For this review, take the finished solid that the model builds, in its own axes (mm). A direction names the side the tool comes from. Give positions to 0.01 mm unless a question says otherwise; leave off trailing zeros. Loops run counter-clockwise (first coordinate to the right, second up) from the corner with the lowest first, then second, coordinate; pieces in that order, holes last. Notation, with made-up numbers: (27.25, 69) -> (64.25, 69) arc R17 cw to (64.25, 76) -> close; hole circle Ø5 at (33.25, 61.5). An arc over 180 degrees is marked (long way). Answer as CSV lines item,"result". Start each with the question number.
Item 1: The part is to be moulded in two halves that separate along Y. For faces 1 (the face through (-6, -27.695, 57)), 2 (the face through (0, -41, 48.58)), 3 (the face through (5, -29.195, 35)), say which applies: +Y half, -Y half, draft (parallel to the pull), parting line (faces both ways), or undercut.
Item 2: Machinability: for faces 4 (the face through (0, -54.195, 69)), 5 (the face through (-6, -13.445, 6)), 6 (the face through (5, -29.195, 69)), which of the approach directions +Z, -Z, +X, -X, +Y, -Y give a long, thin tool a straight path to every point of the face, cutting with its end or side? Answer none if there is none.
Item 3: Clearance check with flat-ended pins moving along their axes: P1, Ø4.5, axis at y = 16.5, z = 34.5, coming from the +X side; P2, Ø5, axis at y = 9.5, z = 65.5, coming from the +X side; P3, Ø21, axis at y = 1.86, z = 46.03, coming from the +X side. State where each tip first meets the part, or that it passes through.
Item 4: Add section B-B on z = 12. State the section outline as (x, y) points, plus the area to 3 significant figures.
Item 5: Add section A-A on z = 46.03. State the section outline as (x, y) points.
Item 6: Add section C-C on y = -10. State the section outline as (x, z) points.
Item 7: Add section D-D on y = 25.5. State the section outline as (x, z) points, plus the area to 3 significant figures.
Item 8: For L1, parallel to Y at x = -1.25, z = 33; L2, parallel to Z at x = -7.5, y = -44.5; L3, parallel to Z at x = -2, y = -33.5, list the stretches that pass through material, from the lowest coordinate up. Write a range as from..to.
```python
from build123d import *

# Parameters (mm, degrees)
PROFILEEXTRUDE_DEPTH    = 73.76
HOSEWINDOW_W            = 16.29
HOSEWINDOW_H            = 26.5
HOSEWINDOWCUT_DEPTH     = 23.11
CAGESCREWS_R            = 2.4
CAGESCREWSCUT_DEPTH     = 23.11
AXLEHOLECUT_DEPTH       = 23.11
SETSCREWHOLES_R         = 1.539432213
SETSCREWHOLES_R_2       = 1.628953018
SETSCREWHOLESCUT_DEPTH  = 23.11
VELOCITYWINDOW_W        = 12.61
VELOCITYWINDOW_H        = 22.29
VELOCITYWINDOWCUT_DEPTH = 23.11
FILLET3_R               = 7
TRIGGERRACKSLOTCUT_W    = 6.7
TRIGGERRACKSLOTCUT_H    = 6.7
RACKSLOTCUT_DEPTH       = 23.11
FILLET4_R               = 1


with BuildPart() as part:
    # Profile → ProfileExtrude (new body)
    with BuildSketch(Plane.XY):
        with BuildLine():
            Line((10.261269376, -54.194713793), (10.261269376, -29.194713793))
            Line((10.261269376, -29.194713793), (-0.848730624, -29.194713793))
            Line((-0.848730624, -29.194713793), (-0.848730624, -13.194713793))
            ThreePointArc((-0.848730624, -13.194713793), (-4.204080189, -9.618555822), (-6.340730624, -5.204713793))
            Line((-6.340730624, -5.204713793), (-8.928730624, -5.204713793))
            Line((-8.928730624, -5.204713793), (-8.928730624, 6.495286207))
            Line((-8.928730624, 6.495286207), (-6.509650624, 6.495286207))
            ThreePointArc((-6.509650624, 6.495286207), (-4.40075771, 10.230064383), (-1.388730624, 13.283536207))
            Line((-1.388730624, 13.283536207), (-1.388730624, 21.845286207))
            Line((-1.388730624, 21.845286207), (10.261269376, 21.845286207))
            Line((10.261269376, 21.845286207), (10.261269376, 31.845286207))
            Line((10.261269376, 31.845286207), (-11.848730624, 31.845286207))
            Line((-11.848730624, 31.845286207), (-11.848730624, -54.194713793))
            Line((-11.848730624, -54.194713793), (10.261269376, -54.194713793))
        make_face()
    extrude(amount=PROFILEEXTRUDE_DEPTH)

    # HoseWindow → HoseWindowCut (cut, through all)
    with BuildSketch(Plane.ZY.offset(11.848730624)):
        with Locations((56.725, -40.944713793)):
            Rectangle(HOSEWINDOW_W, HOSEWINDOW_H)
    extrude(amount=-HOSEWINDOWCUT_DEPTH, mode=Mode.SUBTRACT)

    # CageScrews → CageScrewsCut (cut, through all)
    with BuildSketch(Plane.ZY.offset(11.848730624)):
        with Locations((7.5, 26.845286207)):
            Circle(CAGESCREWS_R)
        with Locations((66.26, 26.845286207)):
            Circle(CAGESCREWS_R)
        with Locations((7.5, -49.194713793)):
            Circle(CAGESCREWS_R)
        with Locations((69.31, -49.194713793)):
            Circle(CAGESCREWS_R)
    extrude(amount=-CAGESCREWSCUT_DEPTH, mode=Mode.SUBTRACT)

    # AxleHole → AxleHoleCut (cut, through all)
    with BuildSketch(Plane.ZY.offset(11.848730624)):
        with BuildLine():
            Line((47.361, 8.359497151), (47.361, 6.740497151))
            Line((47.361, 6.740497151), (44.699, 6.740497151))
            Line((44.699, 6.740497151), (44.699, 8.359497151))
            ThreePointArc((44.699, 8.359497151), (46.03, -4.783713793), (47.361, 8.359497151))
        make_face()
    extrude(amount=-AXLEHOLECUT_DEPTH, mode=Mode.SUBTRACT)

    # SetScrewHoles → SetScrewHolesCut (cut, through all)
    with BuildSketch(Plane.ZY.offset(11.848730624)):
        with Locations((6.03, 1.855286207)):
            Circle(SETSCREWHOLES_R)
        with Locations((68.03, 1.855286207)):
            Circle(SETSCREWHOLES_R_2)
    extrude(amount=-SETSCREWHOLESCUT_DEPTH, mode=Mode.SUBTRACT)

    # VelocityWindow → VelocityWindowCut (cut, through all)
    with BuildSketch(Plane.ZY.offset(11.848730624)):
        with Locations((32.655, -15.499713793)):
            Rectangle(VELOCITYWINDOW_W, VELOCITYWINDOW_H)
    extrude(amount=-VELOCITYWINDOWCUT_DEPTH, mode=Mode.SUBTRACT)

    # Fillet3
    fillet3_edges = [part.edges().sort_by_distance(p)[0] for p in [
        (-11.848730624, -26.644713793, 32.655),
    ]]
    fillet(fillet3_edges, radius=FILLET3_R)

    # TriggerRackSlotCut → RackSlotCut (cut, through all)
    with BuildSketch(Plane.ZY.offset(11.848730624)):
        with Locations((18.35, -44.494713793)):
            Rectangle(TRIGGERRACKSLOTCUT_W, TRIGGERRACKSLOTCUT_H)
        with Locations((30.95, -44.494713793)):
            Rectangle(TRIGGERRACKSLOTCUT_W, TRIGGERRACKSLOTCUT_H)
        with Locations((5.75, -31.794713793)):
            Rectangle(TRIGGERRACKSLOTCUT_W, TRIGGERRACKSLOTCUT_H)
        with Locations((18.35, -31.794713793)):
            Rectangle(TRIGGERRACKSLOTCUT_W, TRIGGERRACKSLOTCUT_H)
        with Locations((5.75, -16.794713793)):
            Rectangle(TRIGGERRACKSLOTCUT_W, TRIGGERRACKSLOTCUT_H)
        with Locations((18.35, -16.794713793)):
            Rectangle(TRIGGERRACKSLOTCUT_W, TRIGGERRACKSLOTCUT_H)
    extrude(amount=-RACKSLOTCUT_DEPTH, mode=Mode.SUBTRACT)

    # Fillet4
    fillet4_edges = [part.edges().sort_by_distance(p)[0] for p in [
        (-11.848730624, -11.174713793, 73.76),
        (-11.848730624, -18.999713793, 26.35),
        (-11.848730624, -18.999713793, 38.96),
        (-11.848730624, -4.354713793, 32.655),
        (-11.848730624, -44.494713793, 15),
        (-11.848730624, -47.844713793, 18.35),
        (-11.848730624, -44.494713793, 21.7),
        (-11.848730624, -41.144713793, 18.35),
        (-11.848730624, -11.174713793, 0),
        (-11.848730624, -44.494713793, 27.6),
        (-11.848730624, -47.844713793, 30.95),
        (-11.848730624, -44.494713793, 34.3),
        (-11.848730624, -41.144713793, 30.95),
        (-11.848730624, -31.794713793, 2.4),
        (-11.848730624, -35.144713793, 5.75),
        (-11.848730624, -31.794713793, 9.1),
        (-11.848730624, -28.444713793, 5.75),
        (-11.848730624, -31.794713793, 15),
        (-11.848730624, -35.144713793, 18.35),
        (-11.848730624, -31.794713793, 21.7),
        (-11.848730624, -28.444713793, 18.35),
        (-11.848730624, -16.794713793, 2.4),
        (-11.848730624, -20.144713793, 5.75),
        (-11.848730624, -16.794713793, 9.1),
        (-11.848730624, -13.444713793, 5.75),
        (-11.848730624, -54.194713793, 69.315),
        (-11.848730624, 31.845286207, 36.88),
        (-11.848730624, -16.794713793, 15),
        (-11.848730624, -20.144713793, 18.35),
        (-11.848730624, -16.794713793, 21.7),
        (-11.848730624, -13.444713793, 18.35),
        (-11.848730624, -54.194713793, 24.29),
        (-11.848730624, -40.944713793, 64.87),
        (-11.848730624, -27.694713793, 56.725),
        (-11.848730624, -40.944713793, 48.58),
    ]]
    fillet(fillet4_edges, radius=FILLET4_R)


solid = part.part
```
Computed values:
1,face 1,"-Y half"
1,face 2,"draft"
1,face 3,"undercut"
2,face 4,"+Z, -Z, +X, -X, -Y"
2,face 5,"+X, -X"
2,face 6,"+Z, -Z, +X"
3,P1,"x = -1.39"
3,P2,"x = -2.85"
3,P3,"x = -2.48"
4,outline,"(-11.85, -53.19) arc R1 ccw to (-10.85, -54.19) -> (10.26, -54.19) -> (10.26, -29.19) -> (-0.85, -29.19) -> (-0.85, -13.19) arc R16.26 cw to (-6.34, -5.2) -> (-8.93, -5.2) -> (-8.93, 6.5) -> (-6.51, 6.5) arc R16.26 cw to (-1.39, 13.28) -> (-1.39, 21.85) -> (10.26, 21.85) -> (10.26, 31.85) -> (-10.85, 31.85) arc R1 ccw to (-11.85, 30.85) -> close"
4,area,"1,180 mm²"
5,outline,"(-11.85, -53.19) arc R1 ccw to (-10.85, -54.19) -> (10.26, -54.19) -> (10.26, -29.19) -> (-0.85, -29.19) -> (-0.85, -13.19) arc R16.26 cw to (-6.34, -5.2) -> (-8.93, -5.2) -> (-8.93, -4.78) -> (-11.85, -4.78) -> close; (-11.85, 6.74) -> (-6.41, 6.74) arc R16.26 cw to (-1.39, 13.28) -> (-1.39, 21.85) -> (10.26, 21.85) -> (10.26, 31.85) -> (-10.85, 31.85) arc R1 ccw to (-11.85, 30.85) -> close"
6,outline,"(-11.85, 1) arc R1 ccw to (-10.85, 0) -> (-3.93, 0) -> (-3.93, 26.35) -> (-10.85, 26.35) arc R1 ccw to (-11.85, 25.35) -> close; (-11.85, 39.96) arc R1 ccw to (-10.85, 38.96) -> (-3.93, 38.96) -> (-3.93, 73.76) -> (-10.85, 73.76) arc R1 ccw to (-11.85, 72.76) -> close"
7,outline,"(-11.85, 1) arc R1 ccw to (-10.85, 0) -> (10.26, 0) -> (10.26, 5.51) -> (-11.85, 5.51) -> close; (-11.85, 9.49) -> (10.26, 9.49) -> (10.26, 64.27) -> (-11.85, 64.27) -> close; (-11.85, 68.25) -> (10.26, 68.25) -> (10.26, 73.76) -> (-10.85, 73.76) arc R1 ccw to (-11.85, 72.76) -> close"
7,area,"1,450 mm²"
8,L1,"-54.19..-47.84, -41.14..-26.64, 21.85..31.85"
8,L2,"0..15, 21.7..27.6, 34.3..48.58, 64.87..73.76"
8,L3,"0..2.4, 9.1..15, 21.7..48.58, 64.87..73.76"
